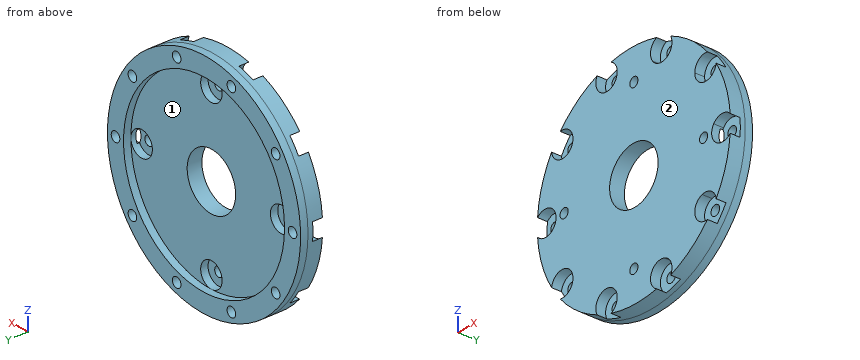
Autodesk Inventor part; units mm, degrees
ref_plane "YZ Plane" through (0, 0, 0) normal (1, 0, 0) x (0, 1, 0)
ref_plane "XZ Plane" through (0, 0, 0) normal (0, 1, 0) x (-1, 0, 0)
ref_plane "XY Plane" through (0, 0, 0) normal (0, 0, 1) x (1, 0, 0)
sketch "Эскиз1" plane through (0, 0, 0) normal (0, 1, 0) x (-1, 0, 0)
  circle A0 centre (0, 0) radius 45
  circle A1 centre (0, 0) radius 37.5
  dimension "d0" = 90
  dimension "d1" = 75
extrude "Выдавливание1" add sketch "Эскиз1" along normal blind 3
sketch "Эскиз2" plane through (0, 0, 0) normal (0, -1, 0) x (1, 0, 0)
  circle A0 centre (0, 0) radius 45
  circle A1 centre (0, 0) radius 45
  circle A2 centre (0, 0) radius 40
  dimension "d4" = 80
  dimension "d5" = 90
extrude "Выдавливание2" add sketch "Эскиз2" along normal blind 6 contours A0 | A2
sketch "Эскиз3" plane through (0, 3, 0) normal (0, 1, 0) x (1, 0, 0)
  circle A0 centre (0, 0) radius 37.5
  circle A1 centre (0, 0) radius 45
  circle A2 centre (41.245, 0) radius 2
  line L0 (37.5, 0) -> (37.9725, 0)
  dimension "d10" = 4
  dimension "d30" = 3.745
extrude "Выдавливание3" cut sketch "Эскиз3" against normal through all contours A2
pattern_circular "Круговой массив1" count 10 over 360 about axis through (0, 0, 0) along (0, 1, 0) of "Выдавливание3"
sketch "Эскиз4" plane through (0, -6, 0) normal (0, -1, 0) x (1, 0, 0)
  circle A0 centre (-33.3679, -24.2432) radius 2
  circle A1 centre (-33.3679, -24.2432) radius 5
  point P0 (0, 0)
  dimension "d16" = 10
extrude "Выдавливание4" cut sketch "Эскиз4" against normal blind 4
pattern_circular "Круговой массив2" count 10 over 360 about axis through (0, 0, 0) along (0, 1, 0) of "Выдавливание4"
sketch "Эскиз5" plane through (0, 0, 0) normal (0, 1, 0) x (1, 0, 0)
  line L0 (15, -27.5) -> (5, -37.5)
  line L1 (5, -37.5) -> (-5, -37.5)
  line L2 (-5, -37.5) -> (-15, -27.5)
  line L3 (-15, -27.5) -> (-27.5, -27.5)
  line L4 (-27.5, -27.5) -> (-27.5, -15)
  line L5 (-27.5, -15) -> (-37.5, -5)
  line L6 (-37.5, -5) -> (-37.5, 5)
  line L7 (-37.5, 5) -> (-27.5, 15)
  line L8 (-27.5, 15) -> (-27.5, 27.5)
  line L9 (-27.5, 27.5) -> (-15, 27.5)
  line L10 (-15, 27.5) -> (-5, 37.5)
  line L11 (-5, 37.5) -> (5, 37.5)
  line L12 (5, 37.5) -> (15, 27.5)
  line L13 (15, 27.5) -> (27.5, 27.5)
  line L14 (27.5, 27.5) -> (27.5, 15)
  line L15 (27.5, 15) -> (37.5, 5)
  line L16 (37.5, 5) -> (37.5, -5)
  line L17 (37.5, -5) -> (27.5, -15)
  line L18 (27.5, -15) -> (27.5, -27.5)
  line L19 (27.5, -27.5) -> (15, -27.5)
  circle A0 centre (0, -32.5) radius 1.9
  circle A1 centre (-32.5, 0) radius 1.9
  circle A2 centre (0, 32.5) radius 1.9
  circle A3 centre (32.5, 0) radius 1.9
  arc A4 (20.5, 15.5) -> (15.5, 20.5) centre (15.5, 15.5) ccw
  arc A5 (15.5, 20.5) -> (10.5, 15.5) centre (15.5, 15.5) ccw
  arc A6 (10.5, 15.5) -> (15.5, 10.5) centre (15.5, 15.5) ccw
  arc A7 (15.5, 10.5) -> (20.5, 15.5) centre (15.5, 15.5) ccw
  arc A8 (-10.5, -15.5) -> (-15.5, -10.5) centre (-15.5, -15.5) ccw
  arc A9 (-15.5, -10.5) -> (-20.5, -15.5) centre (-15.5, -15.5) ccw
  arc A10 (-20.5, -15.5) -> (-15.5, -20.5) centre (-15.5, -15.5) ccw
  arc A11 (-15.5, -20.5) -> (-10.5, -15.5) centre (-15.5, -15.5) ccw
  arc A12 (-10.5, 15.5) -> (-15.5, 20.5) centre (-15.5, 15.5) ccw
  arc A13 (-15.5, 20.5) -> (-20.5, 15.5) centre (-15.5, 15.5) ccw
  arc A14 (-20.5, 15.5) -> (-15.5, 10.5) centre (-15.5, 15.5) ccw
  arc A15 (-15.5, 10.5) -> (-10.5, 15.5) centre (-15.5, 15.5) ccw
  arc A16 (20.5, -15.5) -> (15.5, -10.5) centre (15.5, -15.5) ccw
  arc A17 (15.5, -10.5) -> (10.5, -15.5) centre (15.5, -15.5) ccw
  arc A18 (10.5, -15.5) -> (15.5, -20.5) centre (15.5, -15.5) ccw
  arc A19 (15.5, -20.5) -> (20.5, -15.5) centre (15.5, -15.5) ccw
  arc A20 (11.3, 0) -> (0, 11.3) centre (0, 0) ccw
  arc A21 (0, 11.3) -> (-11.3, 0) centre (0, 0) ccw
  arc A22 (-11.3, 0) -> (0, -11.3) centre (0, 0) ccw
  arc A23 (0, -11.3) -> (11.3, 0) centre (0, 0) ccw
extrude "Выдавливание5" cut sketch "Эскиз5" against normal through all contours A0 | A1 | A2 | A3 | A23 A22 A21 A20
sketch "Эскиз6" plane through (0, 0, 0) normal (0, 1, 0) x (1, 0, 0)
  circle A0 centre (32.5, 0) radius 1.9
  circle A1 centre (32.5, 0) radius 5
  point P0 (0, 0)
  dimension "d24" = 10
extrude "Выдавливание6" cut sketch "Эскиз6" against normal blind 3
pattern_circular "Круговой массив3" count 4 over 360 about axis through (0, 0, 0) along (0, -1, 0) of "Выдавливание6"
properties part number "МД.001.201 - Основа" material "Пластик АБС"
Read the model definition and answer for the solid it produces. Units are mm, in the model's axes. Face numbers are marked on the shaded views. Give positions to 0.01 mm unless a question says otherwise; leave off trailing zeros. Order: outer loops, then holes, each group sorted by start corner. A loop starts at its lowest first (then second) coordinate and runs counter-clockwise, first axis right, second up.
(1) Find section C-C (x = -23.5). Give the vertices of the cut face in (y, z).
(2) Straight lines are drawn through the part: L1, parallel to X at y = 1.5, z = 0 (3 decimals); L2, parallel to Z at x = 12.5, y = -0.75; L3, parallel to Z at x = 2.5, y = -0.75. For each, find the intervals that lie inside material, in ascending order.
(3) For a pull along Z with two mould halves and no side action, classify the marked faces 1 and 2 as released by +Z, released by -Z, zero draft, split by the parting line, or undercut.
(4) Find section A-A (z = 9.5). Give the vertices of the cut face in (x, y), plus the area to 3 significant figures.
(5) Find section D-D (z = 32.5). Give the vertices of the cut face in (x, y), plus the area to 3 significant figures.
(6) Given pin 1 (5 mm diameter, centred on x = -18, y = 1, fed in from -Z); pin 2 (8 mm diameter, centred on x = -12, z = -15, fed in from +Y); pin 3 (3 mm diameter, centred on y = -5, z = -16.5, fed in from -X); pin 4 (3.5 mm diameter, centred on x = -33.37, z = 24.24, fed in from +Y), each flat-ended and moving along its own axis, determine where each tip first touches the part or whether it passes through.
(7) Find section B-B (y = -4.5). Give the vertices of the cut face in (x, z) (3 decimals), plus the area to 3 significant figures.
Result sheet:
1. outline: (-6, -38.38) - (3, -38.38) - (3, -29.22) - (0, -29.22) - (0, 29.22) - (3, 29.22) - (3, 38.38) - (-6, 38.38) - close
2. L1: x = -45 to -43.245, -39.245 to -37.5, 37.5 to 39.245, 43.245 to 45
2. L2: z = -43.23 to -41.21, -37.24 to 37.24, 41.21 to 43.23
2. L3: z = -44.93 to -36.83, -28.17 to -11.02, 11.02 to 28.17, 36.83 to 44.93
3. face 1: undercut
3. face 2: zero draft
4. outline: (-43.99, -6) - (-6.12, -6) - (-6.12, 0) - (-36.28, 0) - (-36.28, 3) - (-43.99, 3) - close; (6.12, -6) - (43.99, -6) - (43.99, 3) - (36.28, 3) - (36.28, 0) - (6.12, 0) - close
4. area: 501 mm2
5. outline: (-31.12, -6) - (-1.9, -6) - (-1.9, -3) - (-5, -3) - (-5, 0) - (-18.71, 0) - (-18.71, 3) - (-31.12, 3) - close; (1.9, -6) - (31.12, -6) - (31.12, 3) - (18.71, 3) - (18.71, 0) - (5, 0) - (5, -3) - (1.9, -3) - close
5. area: 407 mm2
6. pin 1: stops at z = -42.25
6. pin 2: stops at y = 0
6. pin 3: stops at x = -42.43
6. pin 4: passes through
7. outline: (-44.868, -3.446) arc R45 ccw to (-38.324, -23.585) arc R5 cw (long way) to (-34.273, -29.161) arc R45 ccw to (-17.142, -41.607) arc R5 cw (long way) to (-10.588, -43.737) arc R45 ccw to (10.588, -43.737) arc R5 cw (long way) to (17.142, -41.607) arc R45 ccw to (34.273, -29.161) arc R5 cw (long way) to (38.324, -23.585) arc R45 ccw to (44.868, -3.446) arc R5 cw (long way) to (44.868, 3.446) arc R45 ccw to (38.324, 23.585) arc R5 cw (long way) to (34.273, 29.161) arc R45 ccw to (17.142, 41.607) arc R5 cw (long way) to (10.588, 43.737) arc R45 ccw to (-10.588, 43.737) arc R5 cw (long way) to (-17.142, 41.607) arc R45 ccw to (-34.273, 29.161) arc R5 cw (long way) to (-38.324, 23.585) arc R45 ccw to (-44.868, 3.446) arc R5 cw (long way) to start; hole circle Ø3.8 at (-32.5, 0); hole circle Ø22.6 at (0, 0); hole circle Ø3.8 at (0, -32.5); hole circle Ø3.8 at (0, 32.5); hole circle Ø3.8 at (32.5, 0)
7. area: 5,190 mm2
